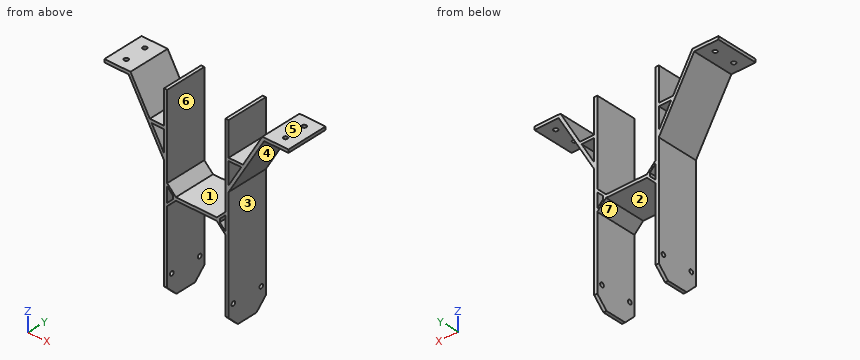
from build123d import *

# Parameters (mm, degrees)
SALIENTE_EXTRUIR1_DEPTH = 40
CROQUIS2_R              = 2
CORTAR_EXTRUIR1_DEPTH   = 155.645237674
CHAFL_N1_SIZE           = 10
CROQUIS3_R              = 2
CORTAR_EXTRUIR2_DEPTH   = 202.82259614


with BuildPart() as part:
    # Croquis1 → Saliente-Extruir1 (new body)
    with BuildSketch(Plane(origin=(0, 0, 0), x_dir=(1, 0, 0), z_dir=(0, 1, 0))):
        Polygon((-28, 9.865463386), (-19.634536614, 1.5), (19.634536614, 1.5), (28, 9.865463386), (28, 90), (31, 90), (31, -28.243932152), (65.068681447, -87), (88.33663064, -87), (88.33663064, -90), (63.33663064, -90), (44.669393136, -57.667396206), (31, -57.667396206), (31, -90), (28, -90), (28, -9.865463386), (19.634536614, -1.5), (-19.634536614, -1.5), (-28, -9.865463386), (-28, -90), (-31, -90), (-31, -57.856759015), (-44.669393136, -57.856759015), (-63.227301971, -90), (-88.227301971, -90), (-88.227301971, -87), (-64.959352778, -87), (-31, -28.180675596), (-31, 90), (-28, 90), align=None)
        Polygon((-28, -7.037036261), (-22.454974268, -1.492010529), (-22.454974268, 1.492010529), (-28, 7.037036261), align=None, mode=Mode.SUBTRACT)
        Polygon((28, -7.011712537), (22.454974268, -1.466686806), (22.454974268, 1.466686806), (28, 7.011712537), align=None, mode=Mode.SUBTRACT)
        Polygon((31, -33.991312786), (43.046670997, -54.856759015), (31, -54.856759015), align=None, mode=Mode.SUBTRACT)
        Polygon((-31, -34.180675596), (-42.937342328, -54.856759015), (-31, -54.856759015), align=None, mode=Mode.SUBTRACT)
    extrude(amount=SALIENTE_EXTRUIR1_DEPTH)

    # Croquis2 → Cortar-Extruir1 (cut, through all)
    with BuildSketch(Plane(origin=(31, 0, 0), x_dir=(0, 0, -1), z_dir=(1, 0, 0))):
        with Locations((70, 35)):
            Circle(CROQUIS2_R)
        with Locations((70, 5)):
            Circle(CROQUIS2_R)
    extrude(amount=-CORTAR_EXTRUIR1_DEPTH, mode=Mode.SUBTRACT)

    # Chaflán1
    chafl_n1_edges = [part.edges().sort_by_distance(p)[0] for p in [
        (29.5, 40, -90),
        (-29.5, 40, -90),
        (29.5, 0, -90),
        (-29.5, 0, -90),
    ]]
    chamfer(chafl_n1_edges, length=CHAFL_N1_SIZE)

    # Croquis3 → Cortar-Extruir2 (cut, through all)
    with BuildSketch(Plane(origin=(0, 0, 87), x_dir=(-1, 0, 0), z_dir=(0, 0, -1))):
        with Locations((-76.702656044, 30)):
            Circle(CROQUIS3_R)
        with Locations((-76.702656044, 10)):
            Circle(CROQUIS3_R)
        with Locations((76.227301971, 30)):
            Circle(CROQUIS3_R)
        with Locations((76.227301971, 10)):
            Circle(CROQUIS3_R)
    extrude(amount=-CORTAR_EXTRUIR2_DEPTH, mode=Mode.SUBTRACT)


solid = part.part
Build history of the part. All positions in model axes, mm. Face numbers are marked on the shaded views. A direction names the side the tool comes from. Give positions to 0.01 mm unless a question says otherwise; leave off trailing zeros. Order: outer loops, then holes, each group sorted by start corner. A loop starts at its lowest first (then second) coordinate and runs counter-clockwise, first axis right, second up. Notation, with made-up numbers: M 43,1 L 100,1 A30 ccw 100,29 Z; hole C 70,31 d11. An arc over 180 degrees is marked long. Use one line per item in the form item = value.
1) Saw through at C-C (z = 71). Give the cut face in (x, y).
Calculated:
outline = M -55.72,0 L -52.26,0 L -52.26,40 L -55.72,40 Z; M -31,0 L -28,0 L -28,40 L -31,40 Z; M 28,0 L 31,0 L 31,40 L 28,40 Z; M 52.37,0 L 55.79,0 L 55.79,40 L 52.37,40 Z
2) Tool access for the marked faces 1, 2 and 3: list every direction of +Z, -Z, +X, -X, +Y, -Y with a clear straight run to the whole face (end or side of a thin tool).
Calculated:
face_1 = +Z, +Y, -Y
face_2 = -Z, +Y, -Y
face_3 = -Z, +X, +Y, -Y
3) Saw through at B-B (x = -15). Give the cut face in (y, z), plus the area to 3 significant figures.
Calculated:
outline = M 0,-1.5 L 40,-1.5 L 40,1.5 L 0,1.5 Z
area = 120 mm2
4) Probe probe 1 along X at (y, z) = (9, -76); probe 2 along X at (y, z) = (25.5, -6.5); probe 3 along X at (y, z) = (7, 58). List the from-to ranges inside material, lowest first.
Calculated:
probe_1 = -31 to -28, 28 to 31
probe_2 = -31 to -28, -27.46 to -24.63, 24.63 to 27.49, 28 to 31
probe_3 = -48.22 to -44.75, -31 to -28, 28 to 31, 44.86 to 48.25
5) Drop flat-ended pins along their axis: pin 1 (3.5 mm diameter, centred on y = 35, z = -70, fed in from +X); pin 2 (1.5 mm diameter, centred on y = 24.5, z = 0, fed in from -X); pin 3 (11 mm diameter, centred on x = 39.5, y = 15.5, fed in from +Z); pin 4 (13.5 mm diameter, centred on x = 34.5, y = 12.5, fed in from -Z). Give the stop position or say it passes through.
Calculated:
pin_1 = through
pin_2 = -31
pin_3 = 58.24
pin_4 = -90
6) Saw through at A-A (z = 25.5). Give the cut face in (x, y).
Calculated:
outline = M -31,0 L -28,0 L -28,40 L -31,40 Z; M 28,0 L 31,0 L 31,40 L 28,40 Z
7) Two-plate mould, pull along X, no slides. Class the marked faces 4, 5, 6 and 7: released by +X, released by -X, zero draft, split by the parting line, or undercut.
Calculated:
face_4 = released by +X
face_5 = zero draft
face_6 = undercut
face_7 = undercut
8) Saw through at D-D (x = 54.5). Give the cut face in (y, z), plus the area to 3 significant figures.
Calculated:
outline = M 0,68.77 L 40,68.77 L 40,74.69 L 0,74.69 Z
area = 237 mm2
